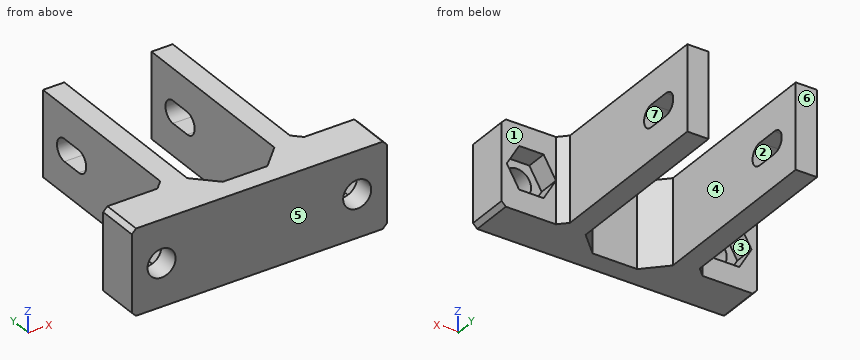
```python
from build123d import *

# Parameters (mm, degrees)
SKETCH2_W           = 60
SKETCH2_H           = 20
SKETCH2_R           = 3.3
BOSS_EXTRUDE2_DEPTH = 5
SKETCH3_W           = 5
SKETCH3_H           = 48
BOSS_EXTRUDE3_DEPTH = 20
CUT_EXTRUDE1_REACH  = 72.403
SKETCH5_W           = 14.75
SKETCH5_H           = 20
BOSS_EXTRUDE4_DEPTH = 5
CHAMFER1_SIZE       = 2
CHAMFER2_SIZE       = 5
CHAMFER3_SIZE       = 1


with BuildPart() as part:
    # Sketch2 → Boss-Extrude2 (new body)
    with BuildSketch(Plane(origin=(0, 0, 0), x_dir=(1, 0, 0), z_dir=(0, 1, 0))):
        Rectangle(SKETCH2_W, SKETCH2_H)
        with Locations(Location((-23, 0, 0), (0, 0, 270))):
            Circle(SKETCH2_R, mode=Mode.SUBTRACT)
        with Locations(Location((23, 0, 0), (0, 0, 270))):
            Circle(SKETCH2_R, mode=Mode.SUBTRACT)
    extrude(amount=BOSS_EXTRUDE2_DEPTH)

    # Sketch3 → Boss-Extrude3 (add)
    with BuildSketch(Plane.XY.offset(10)):
        with Locations((-12.75, 29)):
            Rectangle(SKETCH3_W, SKETCH3_H)
        with Locations((12.75, 29)):
            Rectangle(SKETCH3_W, SKETCH3_H)
    extrude(amount=-BOSS_EXTRUDE3_DEPTH)

    # Cut-Extrude1: up to this face of the body (flat: up to its plane)
    cut_extrude1_end = Plane(part.part.faces().sort_by_distance((-15.25, 29, 0))[0])
    # Sketch4 → Cut-Extrude1 (cut, up to the picked face)
    with BuildSketch(Plane(origin=(15.25, 0, 0), x_dir=(0, 0, -1), z_dir=(1, 0, 0)), mode=Mode.PRIVATE) as cut_extrude1_sk1:
        with BuildLine():
            Line((2.6, 45.5), (2.6, 40.5))
            ThreePointArc((2.6, 40.5), (0, 37.9), (-2.6, 40.5))
            Line((-2.6, 40.5), (-2.6, 45.5))
            ThreePointArc((-2.6, 45.5), (0, 48.1), (2.6, 45.5))
        make_face()
    cut_extrude1_tool1 = split(extrude(cut_extrude1_sk1.sketch, amount=-CUT_EXTRUDE1_REACH, mode=Mode.PRIVATE), bisect_by=cut_extrude1_end, keep=Keep.BOTH, mode=Mode.PRIVATE)
    add(cut_extrude1_tool1.solids().sort_by(Axis((15.25, 43, 0), (-1, 0, 0)))[0], mode=Mode.SUBTRACT)

    # Sketch5 → Boss-Extrude4 (add)
    # profile 1 of 2: a face of its own
    with BuildSketch(Plane(origin=(0, 5, 0), x_dir=(1, 0, 0), z_dir=(0, 1, 0))):
        with Locations((22.625, 0)):
            Rectangle(SKETCH5_W, SKETCH5_H)
        Polygon((28.773502692, 0), (25.886751346, 5), (20.113248654, 5), (17.226497308, 0), (20.113248654, -5), (25.886751346, -5), align=None, mode=Mode.SUBTRACT)
    # profile 2 of 2: a face of its own
    with BuildSketch(Plane(origin=(0, 5, 0), x_dir=(1, 0, 0), z_dir=(0, 1, 0))):
        with Locations((-22.625, 0)):
            Rectangle(SKETCH5_W, SKETCH5_H)
        Polygon((-17.226497308, 0), (-20.113248654, 5), (-25.886751346, 5), (-28.773502692, 0), (-25.886751346, -5), (-20.113248654, -5), align=None, mode=Mode.SUBTRACT)
    extrude(amount=BOSS_EXTRUDE4_DEPTH)

    # Chamfer1
    # the kernel refuses this chamfer: 2 mm, written as the material it adds along each edge
    with BuildSketch(Plane(origin=(15.25, 10, -10), x_dir=(0.9996219169112968, -0.02749587661058651, 0), z_dir=(0, 0, 1))) as chamfer1_piece_1_section:
        Polygon((CHAMFER1_SIZE * 0.999621916911, CHAMFER1_SIZE * 0.0274958766106), (-CHAMFER1_SIZE * 0.0274958766106, CHAMFER1_SIZE * 0.999621916911), (0, 0), align=None)
    chamfer1_piece_1 = extrude(amount=20, mode=Mode.PRIVATE)
    chamfer1_piece_1 = split(chamfer1_piece_1, bisect_by=Plane(origin=(14.273862805, 10.629145716, -5.114112976), z_dir=(0.8660254037844387, 0, -0.49999999999999994)), keep=Keep.TOP, mode=Mode.PRIVATE)
    chamfer1_piece_1 = split(chamfer1_piece_1, bisect_by=Plane(origin=(19.549147449, 10.629145716, -4.022948051), z_dir=(-0.8660254037844387, 0, -0.49999999999999994)), keep=Keep.TOP, mode=Mode.PRIVATE)
    add(chamfer1_piece_1)
    with BuildSketch(Plane(origin=(15.25, 10, -10), x_dir=(0.9996219169112968, -0.02749587661058651, 0), z_dir=(0, 0, 1))) as chamfer1_piece_2_section:
        Polygon((CHAMFER1_SIZE * 0.999621916911, CHAMFER1_SIZE * 0.0274958766106), (-CHAMFER1_SIZE * 0.0274958766106, CHAMFER1_SIZE * 0.999621916911), (0, 0), align=None)
    chamfer1_piece_2 = extrude(amount=20, mode=Mode.PRIVATE)
    chamfer1_piece_2 = split(chamfer1_piece_2, bisect_by=Plane(origin=(16.849076721, 10.762644927, -0.653711633), z_dir=(-0.8660254037844387, 0, 0.49999999999999994)), keep=Keep.TOP, mode=Mode.PRIVATE)
    chamfer1_piece_2 = split(chamfer1_piece_2, bisect_by=Plane(origin=(16.849076721, 10.762644927, 0.653711633), z_dir=(-0.8660254037844387, 0, -0.49999999999999994)), keep=Keep.TOP, mode=Mode.PRIVATE)
    add(chamfer1_piece_2)
    with BuildSketch(Plane(origin=(15.25, 10, -10), x_dir=(0.9996219169112968, -0.02749587661058651, 0), z_dir=(0, 0, 1))) as chamfer1_piece_3_section:
        Polygon((CHAMFER1_SIZE * 0.999621916911, CHAMFER1_SIZE * 0.0274958766106), (-CHAMFER1_SIZE * 0.0274958766106, CHAMFER1_SIZE * 0.999621916911), (0, 0), align=None)
    chamfer1_piece_3 = extrude(amount=20, mode=Mode.PRIVATE)
    chamfer1_piece_3 = split(chamfer1_piece_3, bisect_by=Plane(origin=(19.549147449, 10.629145716, 4.022948051), z_dir=(-0.8660254037844387, 0, 0.49999999999999994)), keep=Keep.TOP, mode=Mode.PRIVATE)
    chamfer1_piece_3 = split(chamfer1_piece_3, bisect_by=Plane(origin=(14.273862805, 10.629145716, 5.114112976), z_dir=(0.8660254037844387, 0, 0.49999999999999994)), keep=Keep.TOP, mode=Mode.PRIVATE)
    add(chamfer1_piece_3)
    with BuildSketch(Plane(origin=(-15.25, 10, 10), x_dir=(0.027495876610586487, 0.9996219169112968, 0), z_dir=(0, 0, -1))) as chamfer1_piece_4_section:
        Polygon((CHAMFER1_SIZE * 0.999621916911, -CHAMFER1_SIZE * 0.0274958766106), (-CHAMFER1_SIZE * 0.0274958766106, -CHAMFER1_SIZE * 0.999621916911), (0, 0), align=None)
    chamfer1_piece_4 = extrude(amount=20, mode=Mode.PRIVATE)
    chamfer1_piece_4 = split(chamfer1_piece_4, bisect_by=Plane(origin=(-14.273862805, 10.629145716, 5.114112976), z_dir=(-0.8660254037844387, 0, 0.49999999999999994)), keep=Keep.TOP, mode=Mode.PRIVATE)
    chamfer1_piece_4 = split(chamfer1_piece_4, bisect_by=Plane(origin=(-19.549147449, 10.629145716, 4.022948051), z_dir=(0.8660254037844388, 0, 0.49999999999999967)), keep=Keep.TOP, mode=Mode.PRIVATE)
    add(chamfer1_piece_4)
    with BuildSketch(Plane(origin=(-15.25, 10, 10), x_dir=(0.027495876610586487, 0.9996219169112968, 0), z_dir=(0, 0, -1))) as chamfer1_piece_5_section:
        Polygon((CHAMFER1_SIZE * 0.999621916911, -CHAMFER1_SIZE * 0.0274958766106), (-CHAMFER1_SIZE * 0.0274958766106, -CHAMFER1_SIZE * 0.999621916911), (0, 0), align=None)
    chamfer1_piece_5 = extrude(amount=20, mode=Mode.PRIVATE)
    chamfer1_piece_5 = split(chamfer1_piece_5, bisect_by=Plane(origin=(-16.849076721, 10.762644927, 0.653711633), z_dir=(0.8660254037844387, 0, -0.49999999999999994)), keep=Keep.TOP, mode=Mode.PRIVATE)
    chamfer1_piece_5 = split(chamfer1_piece_5, bisect_by=Plane(origin=(-16.849076721, 10.762644927, -0.653711633), z_dir=(0.8660254037844388, 0, 0.49999999999999967)), keep=Keep.TOP, mode=Mode.PRIVATE)
    add(chamfer1_piece_5)
    with BuildSketch(Plane(origin=(-15.25, 10, 10), x_dir=(0.027495876610586487, 0.9996219169112968, 0), z_dir=(0, 0, -1))) as chamfer1_piece_6_section:
        Polygon((CHAMFER1_SIZE * 0.999621916911, -CHAMFER1_SIZE * 0.0274958766106), (-CHAMFER1_SIZE * 0.0274958766106, -CHAMFER1_SIZE * 0.999621916911), (0, 0), align=None)
    chamfer1_piece_6 = extrude(amount=20, mode=Mode.PRIVATE)
    chamfer1_piece_6 = split(chamfer1_piece_6, bisect_by=Plane(origin=(-19.549147449, 10.629145716, -4.022948051), z_dir=(0.8660254037844387, 0, -0.49999999999999994)), keep=Keep.TOP, mode=Mode.PRIVATE)
    chamfer1_piece_6 = split(chamfer1_piece_6, bisect_by=Plane(origin=(-14.273862805, 10.629145716, -5.114112976), z_dir=(-0.8660254037844388, 0, -0.49999999999999967)), keep=Keep.TOP, mode=Mode.PRIVATE)
    add(chamfer1_piece_6)

    # Chamfer2
    chamfer2_edges = [part.edges().sort_by_distance(p)[0] for p in [
        (-10.25, 5, 0),
        (10.25, 5, 0),
    ]]
    chamfer(chamfer2_edges, length=CHAMFER2_SIZE)

    # Chamfer3
    chamfer3_edges = [part.edges().sort_by_distance(p)[0] for p in [
        (30, 5, 10),
        (-30, 5, 10),
        (-30, 5, -10),
        (30, 5, -10),
    ]]
    chamfer(chamfer3_edges, length=CHAMFER3_SIZE)


solid = part.part
```
Verification items for the finished model (mm, model axes). Face numbers are marked on the shaded views. A direction names the side the tool comes from. Coordinates: 2 decimals unless noted, no trailing zeros. Write each loop counter-clockwise with the first axis right and the second up, starting at its lowest first coordinate (ties: lowest second). Pieces come first, ordered by that corner, then holes. Notation, with made-up numbers: M 4.5,-5 L 50.5,-5 A16 ccw 50.5,4 Z; hole C -31.5,51 d6. An arc over 180 degrees is marked long. One line per item, written item: value.
Item 1: Gauge pin test, flat ends, axial feed: pin 1 Ø6.5 at (x, z) = (-26.5, -2) entering from +Y; pin 2 Ø10 at (x, z) = (-4.5, 0) entering from +Y; pin 3 Ø10 at (y, z) = (41, -0.5) entering from +X. Record the tip position at first contact, or that the pin passes through.
Check sheet entries:
pin 1: stops at y = 10
pin 2: stops at y = 9.25
pin 3: stops at x = 15.25
Item 2: Section check D-D, the plane x = -14.5. Record the boundary of the cut face in (y, z), plus the area to 3 significant figures.
Check sheet entries:
outline: M 0,-10 L 53,-10 L 53,10 L 0,10 Z; hole M 40.5,-2.6 L 45.5,-2.6 A2.6 ccw 45.5,2.6 L 40.5,2.6 A2.6 ccw Z
area: 1,010 mm^2
Item 3: Section check C-C, the plane y = 29.5. Record the boundary of the cut face in (x, z), plus the area to 3 significant figures.
Check sheet entries:
outline: M -15.25,-10 L -10.25,-10 L -10.25,10 L -15.25,10 Z; M 10.25,-10 L 15.25,-10 L 15.25,10 L 10.25,10 Z
area: 200 mm^2
Item 4: Scan lines: line 1 along X through (y, z) = (3.7, 0); line 2 along X through (y, z) = (35, -7.25); line 3 along Z through (x, y) = (-10.5, 42.5). Record each from-to range of solid material in increasing order.
Check sheet entries:
line 1: x = -30 to -26.3, -19.7 to 19.7, 26.3 to 30
line 2: x = -15.25 to -10.25, 10.25 to 15.25
line 3: z = -10 to -2.6, 2.6 to 10
Item 5: Mould release check, pull along Y, two halves, no side actions. Record for the marked faces 5, 6 and 7: pulls with the +Y half, pulls with the -Y half, needs draft (parallel to the pull), parting line crosses it, or undercut.
Check sheet entries:
face 5: pulls with the -Y half
face 6: pulls with the +Y half
face 7: undercut
Item 6: Access from +Z, -Z, +X, -X, +Y, -Y to the whole of each face (thin tool, end or side, straight path). Record for the marked faces 1, 2, 3 and 4.
Check sheet entries:
face 1: +Z, -Z, +X, +Y
face 2: +X, -X
face 3: +Y
face 4: +Z, -Z, +Y
Item 7: Section check A-A, the plane y = 6.5. Record the boundary of the cut face in (x, z), plus the area to 3 significant figures.
Check sheet entries:
outline: M -30,-9 L -29,-10 L -6.75,-10 L -6.75,10 L -29,10 L -30,9 Z; M 6.75,-10 L 29,-10 L 30,-9 L 30,9 L 29,10 L 6.75,10 Z; hole M -28.77,0 L -25.89,-5 L -20.11,-5 L -17.23,0 L -20.11,5 L -25.89,5 Z; hole M 17.23,0 L 20.11,-5 L 25.89,-5 L 28.77,0 L 25.89,5 L 20.11,5 Z
area: 755 mm^2
Item 8: Section check B-B, the plane x = -23. Record the boundary of the cut face in (y, z), plus the area to 3 significant figures.
Check sheet entries:
outline: M 0,-10 L 10,-10 L 10,-5 L 5,-5 L 5,-3.3 L 0,-3.3 Z; M 0,3.3 L 5,3.3 L 5,5 L 10,5 L 10,10 L 0,10 Z
area: 117 mm^2
